Design review of the part shown in the three views and the two pictorial views. Dimensions are in mm from the part's minimum x, y and z. Give positions to 0.01 mm unless a question says otherwise; leave off trailing zeros. Write each loop counter-clockwise with the first axis right and the second up, starting at its lowest first coordinate (ties: lowest second). Pieces come first, ordered by that corner, then holes. Notation, with made-up numbers: M 0.25,83 L 43.25,83 A15 ccw 43.25,91 Z; hole C -35,-5 d7. An arc over 180 degrees is marked long. Write item = value, one per line.
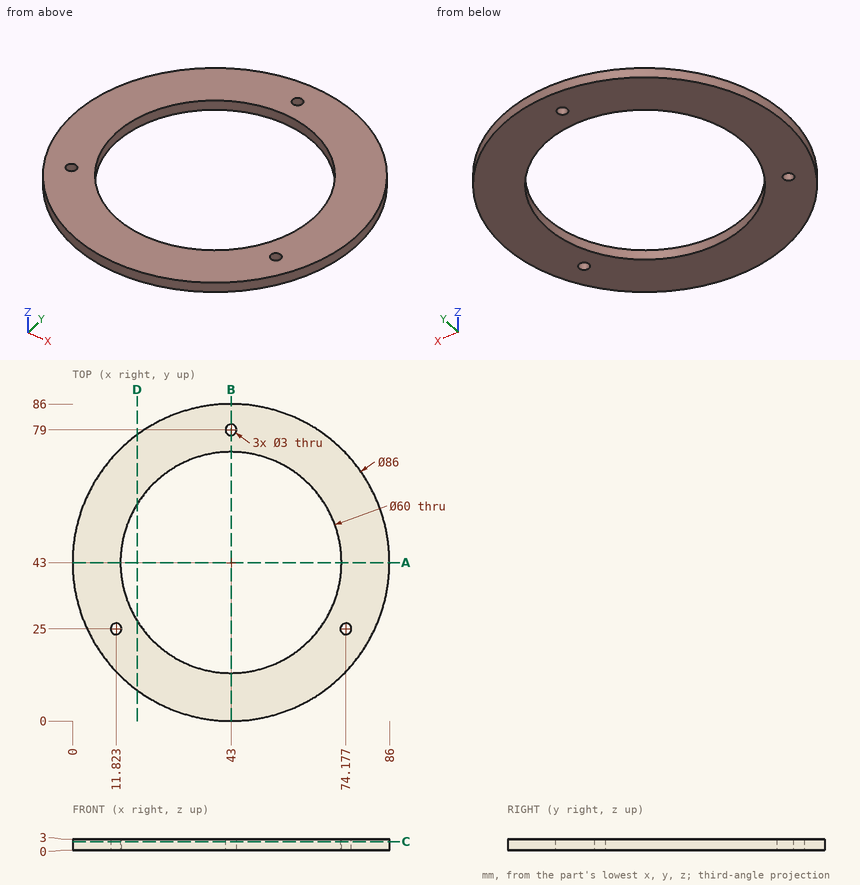
1. For line 1 along Y through (x, z) = (43, 0.5); line 2 along X through (y, z) = (66.5, 1.05); line 3 along X through (y, z) = (62, 1.7) (1 decimal), list the stretches that pass through material, from the lowest coordinate up. Write a range as from..to.
Responses:
line_1 = 0..13, 73..77.5, 80.5..86
line_2 = 6.99..24.35, 61.65..79.01
line_3 = 4.4..19.8, 66.2..81.6
2. Insertion check: P1, Ø4, axis at x = 11.82, y = 25, coming from the +Z side; P2, Ø1, axis at x = 39, z = 1, coming from the +Y side; P3, Ø2.5, axis at x = 43, y = 79, coming from the -Z side. Each pin has a flat end and moves straight along its axis. Give the tip position at first contact, or say it passes through.
Responses:
P1 = 3
P2 = 85.86
P3 = through
3. We need section C-C, the plane z = 2.3. Write out the cut boundary in (x, y).
Responses:
outline = C 43,43 d86; hole C 11.82,25 d3; hole C 43,43 d60; hole C 43,79 d3; hole C 74.18,25 d3
4. We need section A-A, the plane y = 43. Write out the cut boundary in (x, z).
Responses:
outline = M 0,0 L 13,0 L 13,3 L 0,3 Z; M 73,0 L 86,0 L 86,3 L 73,3 Z
5. We need section B-B, the plane x = 43. Write out the cut boundary in (y, z), then the cut area to 3 significant figures.
Responses:
outline = M 0,0 L 13,0 L 13,3 L 0,3 Z; M 73,0 L 77.5,0 L 77.5,3 L 73,3 Z; M 80.5,0 L 86,0 L 86,3 L 80.5,3 Z
area = 69.0 mm2
6. We need section D-D, the plane x = 17.5. Write out the cut boundary in (y, z), then the cut area to 3 significant figures.
Responses:
outline = M 8.38,0 L 27.2,0 L 27.2,3 L 8.38,3 Z; M 58.8,0 L 77.62,0 L 77.62,3 L 58.8,3 Z
area = 113 mm2
